Work out the finished part from the listing and answer in its coordinate system (mm). A direction names the side the tool comes from. Round coordinates to 2 decimals unless told otherwise and drop trailing zeros. Order: outer loops, then holes, each group sorted by start corner. A loop starts at its lowest first (then second) coordinate and runs counter-clockwise, first axis right, second up. Notation, with made-up numbers: (-39.5, 73) - (-10.5, 73) arc R28 cw to (-10.5, 99) - close; hole circle Ø6 at (32, -8). An arc over 180 degrees is marked (long way). Put each result on its own line as item: value.
```python
from build123d import *

# Parameters (mm, degrees)
F1_DEPTH = 2
F0_W     = 8
F0_H     = 5.5
F2_DEPTH = 7.5
F4_DEPTH = 5
F5_DEPTH = 0.5
F6_F1_R  = 1
F6_F2_R  = 1


with BuildPart() as f1:
    # F0 (on Right) → F1 (new body, symmetric)
    with BuildSketch(Plane.YZ):
        Polygon((42, 5.5), (10, 5.5), (0, 0), (42, 0), align=None)
    extrude(amount=F1_DEPTH, both=True)

    # F0 (on Right) → F2 (join, symmetric)
    with BuildSketch(Plane.YZ):
        with Locations((46, 2.75)):
            Rectangle(F0_W, F0_H)
    extrude(amount=F2_DEPTH, both=True)

    # F3 (on face) → F4 (cut)
    with BuildSketch(Plane.XY.offset(5.5)):
        with BuildLine():
            ThreePointArc((-2.75, 48.75), (-5.5, 46), (-2.75, 43.25))
            Line((-2.75, 43.25), (2.75, 43.25))
            ThreePointArc((2.75, 43.25), (5.5, 46), (2.75, 48.75))
            Line((2.75, 48.75), (-2.75, 48.75))
        make_face()
    extrude(amount=-F4_DEPTH, mode=Mode.SUBTRACT)

    # F3 (on face) → F5 (join)
    with BuildSketch(Plane.XY.offset(5.5)):
        with BuildLine():
            ThreePointArc((-2.75, 48.75), (-5.5, 46), (-2.75, 43.25))
            Line((-2.75, 43.25), (2.75, 43.25))
            ThreePointArc((2.75, 43.25), (5.5, 46), (2.75, 48.75))
            Line((2.75, 48.75), (-2.75, 48.75))
        make_face()
    extrude(amount=-F5_DEPTH)

    # F6: fillet of radius 1 on 21 edges, made by hand

    # F6_f1
    f6_f1_edges = [f1.edges().sort_by_distance(p)[0] for p in [
        (2, 42, 2.75),
        (-2, 42, 2.75),
    ]]
    fillet(f6_f1_edges, radius=F6_F1_R)

    # F6_f2
    f6_f2_edges = [f1.edges().sort_by_distance(p)[0] for p in [
        (-7.5, 42, 2.75),
        (-7.5, 50, 2.75),
        (7.5, 50, 2.75),
        (7.5, 42, 2.75),
        (-7.5, 46, 5.5),
        (-5.25, 42, 5.5),
        (-2, 25.5, 5.5),
        (0, 10, 5.5),
        (2, 25.5, 5.5),
        (5.25, 42, 5.5),
        (7.5, 46, 5.5),
        (0, 50, 5.5),
        (2, 5, 2.75),
        (2, 20.5, 0),
        (-2, 5, 2.75),
        (-2, 20.5, 0),
        (0, 50, 0),
        (7.5, 46, 0),
        (-7.5, 46, 0),
        (-2.2928932188, 41.7071067812, 0),
        (2.2928932188, 41.7071067812, 0),
        (2.2928932188, 41.7071067812, 5.5),
        (-2.2928932188, 41.7071067812, 5.5),
    ]]
    fillet(f6_f2_edges, radius=F6_F2_R)


solid = f1.part
```
1) Straight lines are drawn through the part: L1, parallel to Z at x = -1.25, y = 44; L2, parallel to X at y = 12, z = 4.05; L3, parallel to Y at x = 5, z = 1.4. For each, find the intervals that lie inside material, in ascending order. Write a range as from..to.
Findings below:
L1: z = 0..0.5, 5..5.5
L2: x = -2..2
L3: y = 42..44.42, 47.58..50
2) A cutting plane is placed at D-D on x = 3.5. Write down the section's boundary in (y, z), then the cut area to 3 significant figures.
Findings below:
outline: (42, 1) arc R1 ccw to (43, 0) - (49, 0) arc R1 ccw to (50, 1) - (50, 4.5) arc R1 ccw to (49, 5.5) - (43, 5.5) arc R1 ccw to (42, 4.5) - close; hole (43.35, 0.5) - (48.65, 0.5) - (48.65, 5) - (43.35, 5) - close
area: 19.3 mm2
3) For a pull along X with two mould halves and no side action, classify faces 1 (the flat face through (0, 43.25, 3)), 2 (the flat face through (0, 32, 0)), 3 (the flat face through (-7.5, 46, 3)) as pulls with the +X half, pulls with the -X half, needs draft (parallel to the pull), parting line crosses it, or undercut.
Findings below:
face 1: undercut
face 2: needs draft
face 3: pulls with the -X half
4) For faces 4 (the flat face through (-2, 22, 3)), 5 (the cylindrical face through (-4.774, 42.285, 0.301)), 6 (the cylindrical face through (4.774, 42.285, 0.301)), determine the directions among +Z, -Z, +X, -X, +Y, -Y from which every point of the face is accessible in a straight line to the end or side of a thin tool.
Findings below:
face 4: +Z, -Z, -X, -Y
face 5: -Z, -X, -Y
face 6: -Z, +X, -Y
5) A cutting plane is placed at C-C on y = 46. Write down the section's boundary in (x, z).
Findings below:
outline: (-7.5, 1) arc R1 ccw to (-6.5, 0) - (6.5, 0) arc R1 ccw to (7.5, 1) - (7.5, 4.5) arc R1 ccw to (6.5, 5.5) - (-6.5, 5.5) arc R1 ccw to (-7.5, 4.5) - close; hole (-5.5, 0.5) - (5.5, 0.5) - (5.5, 5) - (-5.5, 5) - close
6) Given pin 1 Ø2 at (x, z) = (-5, 4.5) entering from -Y; pin 2 Ø5 at (x, y) = (-2, 27) entering from -Z; pin 3 Ø2 at (x, z) = (0, 2) entering from -Y; pin 4 Ø1 at (y, z) = (20, 3) entering from -X, each flat-ended and moving along its own axis, determine where each tip first touches the part or whether it passes through.
Findings below:
pin 1: stops at y = 42
pin 2: stops at z = 0
pin 3: stops at y = 1.82
pin 4: stops at x = -2
7) A cutting plane is placed at A-A on x = 0. Write down the section's boundary in (y, z).
Findings below:
outline: (0, 0) - (49, 0) arc R1 ccw to (50, 1) - (50, 4.5) arc R1 ccw to (49, 5.5) - (10.26, 5.5) arc R1 ccw to (9.77, 5.38) - close; hole (43.25, 0.5) - (48.75, 0.5) - (48.75, 5) - (43.25, 5) - close
8) A cutting plane is placed at B-B on y = 35. Write down the section's boundary in (x, z), then the cut area to 3 significant figures.
Findings below:
outline: (-2, 1) arc R1 ccw to (-1, 0) - (1, 0) arc R1 ccw to (2, 1) - (2, 4.5) arc R1 ccw to (1, 5.5) - (-1, 5.5) arc R1 ccw to (-2, 4.5) - close
area: 21.1 mm2
